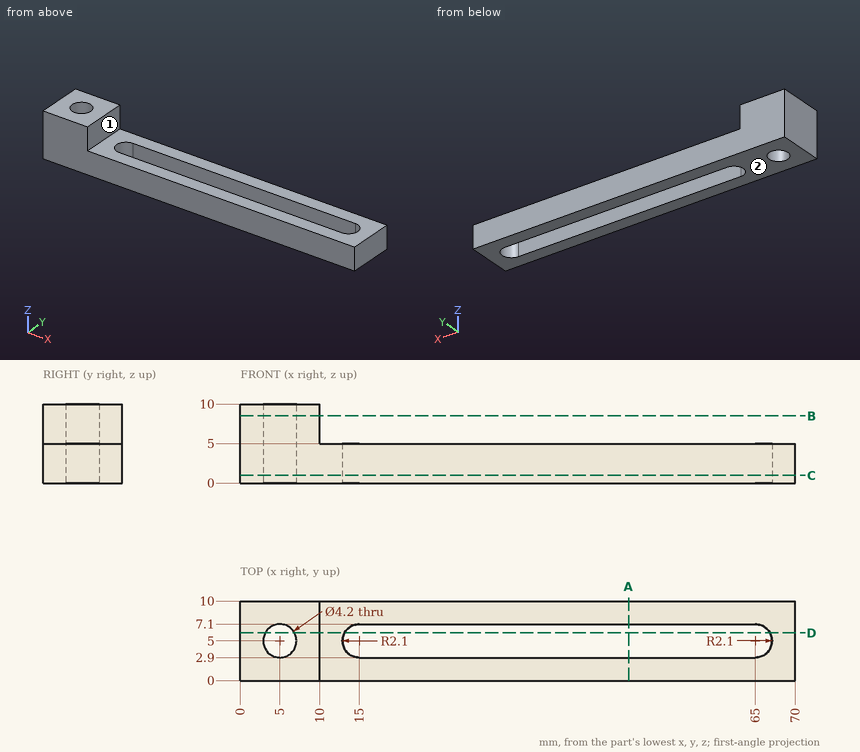
Input: dimensioned drawing with shaded views. Units: mm. Origin: part minimum x, y, z. A direction names the side the tool comes from. Give positions to 0.01 mm unless a question says otherwise; leave off trailing zeros. Write each loop counter-clockwise with the first axis right and the second up, starting at its lowest first coordinate (ties: lowest second). Pieces come first, ordered by that corner, then holes.
Q1. Section A-A, the plane x = 49. Output: boundary loops of the cut face in (y, z), plus the area to 3 significant figures.
Q2. Material intervals for probe 1 along Y at (x, z) = (20, 0.5); probe 2 along X at (y, z) = (6.25, 1.25); probe 3 along X at (y, z) = (5.5, 3.75), sorted ascending.
Q3. Section B-B, the plane z = 8.5. Output: boundary loops of the cut face in (x, y), plus the area to 3 significant figures.
Q4. First-contact query: P1, Ø6, axis at x = 21.5, z = 7, coming from the -Y side; P2, Ø5.5, axis at y = 7.5, z = 8.5, coming from the +X side; P3, Ø6, axis at x = 18, y = 8, coming from the +Z side. Flat tips, straight axial feed; report the tip coordinate or a pass-through.
Q5. Set-up query: the marked faces 1 and 2. Return all of +Z, -Z, +X, -X, +Y, -Y with unobstructed straight access to the full face (end or side cutting, diameter ignored); none if empty.
Q6. Section C-C, the plane z = 1. Output: boundary loops of the cut face in (x, y).
Q7. Section D-D, the plane y = 6. Output: boundary loops of the cut face in (x, z).
Filled in:
1. outline: (0, 0) - (2.9, 0) - (2.9, 5) - (0, 5) - close; (7.1, 0) - (10, 0) - (10, 5) - (7.1, 5) - close
1. area: 29.0 mm2
2. probe 1: y = 0 to 2.9, 7.1 to 10
2. probe 2: x = 0 to 3.31, 6.69 to 13.31, 66.69 to 70
2. probe 3: x = 0 to 2.96, 7.04 to 12.96, 67.04 to 70
3. outline: (0, 0) - (10, 0) - (10, 10) - (0, 10) - close; hole circle Ø4.2 at (5, 5)
3. area: 86.1 mm2
4. P1: stops at y = 0
4. P2: stops at x = 10
4. P3: stops at z = 5
5. face 1: +Z, +X, +Y, -Y
5. face 2: -Z, +X, -X, +Y, -Y
6. outline: (0, 0) - (70, 0) - (70, 10) - (0, 10) - close; hole circle Ø4.2 at (5, 5); hole (15, 2.9) - (65, 2.9) arc R2.1 ccw to (65, 7.1) - (15, 7.1) arc R2.1 ccw to start
7. outline: (0, 0) - (3.15, 0) - (3.15, 10) - (0, 10) - close; (6.85, 0) - (13.15, 0) - (13.15, 5) - (10, 5) - (10, 10) - (6.85, 10) - close; (66.85, 0) - (70, 0) - (70, 5) - (66.85, 5) - close
